from build123d import *

# Parameters (mm, degrees)
SKETCH1_R                = 7.15
SKETCH1_R_2              = 6.65
BOSS_EXTRUDE1_DEPTH      = 15
BOSS_EXTRUDE2_DEPTH      = 26.9
BOSS_EXTRUDE2_DEPTH_BACK = 11.9
SKETCH2_R                = 14
SKETCH2_R_2              = 8.9
CUT_EXTRUDE12_START      = -15
SKETCH50_R               = 14
SKETCH50_R_2             = 10.9
CUT_EXTRUDE12_DEPTH      = 10
CUT_EXTRUDE8_DEPTH       = 10
CUT_EXTRUDE8_DEPTH_BACK  = 21.28
SKETCH30_R               = 7.65
CIRPATTERN3_COUNT        = 6
BOSS_EXTRUDE3_START      = 1.2999999
BOSS_EXTRUDE3_DEPTH      = 1.6000002
CUT_EXTRUDE11_START      = 2.5
SKETCH38_R               = 11.53
CUT_EXTRUDE11_DEPTH      = 10
CUT_EXTRUDE13_DEPTH      = 39.000263325
CUT_EXTRUDE13_DEPTH_BACK = 39.000263325
SKETCH51_W               = 20.008016057
SKETCH51_H               = 32.534282003
CIRPATTERN4_COUNT        = 6
FILLET1_R                = 0.25


# Read off the part's stored shape, not the designer's step: Boss-Extrude3
with BuildPart() as part:
    # Sketch1 → Boss-Extrude1 (new body)
    with BuildSketch(Plane.XY):
        Circle(SKETCH1_R)
        Circle(SKETCH1_R_2, mode=Mode.SUBTRACT)
    extrude(amount=BOSS_EXTRUDE1_DEPTH)

    # Sketch2 → Boss-Extrude2 (add, two sides: drawn at the far end of the back side and taken through both)
    with BuildSketch(Plane(origin=(0, 0, 0), x_dir=(1, 0, 0), z_dir=(0, 1, 0)).offset(-BOSS_EXTRUDE2_DEPTH_BACK)):
        with Locations(Location((0, 8.9, 0), (0, 0, 270))):
            Circle(SKETCH2_R)
        with Locations(Location((0, 8.9, 0), (0, 0, 270))):
            Circle(SKETCH2_R_2, mode=Mode.SUBTRACT)
    extrude(amount=BOSS_EXTRUDE2_DEPTH + BOSS_EXTRUDE2_DEPTH_BACK)

    # Sketch50 → Cut-Extrude12 (cut)
    with BuildSketch(Plane(origin=(0, 26.9, 0), x_dir=(1, 0, 0), z_dir=(0, 1, 0)).offset(CUT_EXTRUDE12_START)):
        with Locations(Location((0, 8.9, 0), (0, 0, 270))):
            Circle(SKETCH50_R)
        with Locations(Location((0, 8.9, 0), (0, 0, 270))):
            Circle(SKETCH50_R_2, mode=Mode.SUBTRACT)
    extrude(amount=CUT_EXTRUDE12_DEPTH, mode=Mode.SUBTRACT)

    # Sketch30 → Cut-Extrude8 (cut, two sides: drawn at the far end of the back side and taken through both)
    with BuildSketch(Plane.XY.offset(15).offset(-CUT_EXTRUDE8_DEPTH_BACK)):
        with Locations(Location((0, 0, 0), (0, 0, 90.000000001))):
            Circle(SKETCH30_R)
    extrude(amount=CUT_EXTRUDE8_DEPTH + CUT_EXTRUDE8_DEPTH_BACK, mode=Mode.SUBTRACT)

    # Sketch47 → Tap Drill for M2 Tap1 (revolve, cut)
    with BuildSketch(Plane(origin=(0, 26.9, 2.1), x_dir=(0, 0, 1), z_dir=(1, 0, 0))):
        Polygon((0, 0), (0, 4.480688495), (0.8, 4), (0.8, 0), align=None)
    tap_drill_for_m2_tap1 = revolve(axis=Axis((0, 33.25, 2.1), (0, -1, 0)), mode=Mode.SUBTRACT)

    # CirPattern3: Tap Drill for M2 Tap1 ×6 about axis
    cirpattern3_axis = Axis((0, 0, -8.9), (0, 1, 0))
    for i in range(1, CIRPATTERN3_COUNT):
        add(tap_drill_for_m2_tap1.rotate(cirpattern3_axis, i * 360 / CIRPATTERN3_COUNT), mode=Mode.SUBTRACT)

    # Mirror1: Tap Drill for M2 Tap1 across plane
    add(tap_drill_for_m2_tap1.mirror(Plane.ZX.offset(7.5)), mode=Mode.SUBTRACT)

    # Mirror1 copy 1 sketch → Mirror1 copy 1 (revolve, cut)
    with BuildSketch(Plane(origin=(9.526279442, -11.9, -3.4), x_dir=(0.8660254037844386, 0, 0.5000000000000001), z_dir=(0.5000000000000001, 0, -0.8660254037844386))):
        Polygon((0, 0), (0, -4.480688495), (0.8, -4), (0.8, 0), align=None)
    revolve(axis=Axis((9.526279442, -18.25, -3.4), (0, -1, 0)), mode=Mode.SUBTRACT)

    # Mirror1 copy 2 sketch → Mirror1 copy 2 (revolve, cut)
    with BuildSketch(Plane(origin=(9.526279442, -11.9, -14.4), x_dir=(0.8660254037844387, 0, -0.4999999999999998), z_dir=(-0.4999999999999998, 0, -0.8660254037844387))):
        Polygon((0, 0), (0, -4.480688495), (0.8, -4), (0.8, 0), align=None)
    revolve(axis=Axis((9.526279442, -18.25, -14.4), (0, -1, 0)), mode=Mode.SUBTRACT)

    # Mirror1 copy 3 sketch → Mirror1 copy 3 (revolve, cut)
    with BuildSketch(Plane(origin=(0, -11.9, -19.9), x_dir=(0, 0, -1), z_dir=(-1, 0, 0))):
        Polygon((0, 0), (0, -4.480688495), (0.8, -4), (0.8, 0), align=None)
    revolve(axis=Axis((0, -18.25, -19.9), (0, -1, 0)), mode=Mode.SUBTRACT)

    # Mirror1 copy 4 sketch → Mirror1 copy 4 (revolve, cut)
    with BuildSketch(Plane(origin=(-9.526279442, -11.9, -14.4), x_dir=(-0.8660254037844384, 0, -0.5000000000000004), z_dir=(-0.5000000000000004, 0, 0.8660254037844384))):
        Polygon((0, 0), (0, -4.480688495), (0.8, -4), (0.8, 0), align=None)
    revolve(axis=Axis((-9.526279442, -18.25, -14.4), (0, -1, 0)), mode=Mode.SUBTRACT)

    # Mirror1 copy 5 sketch → Mirror1 copy 5 (revolve, cut)
    with BuildSketch(Plane(origin=(-9.526279442, -11.9, -3.4), x_dir=(-0.8660254037844386, 0, 0.5000000000000001), z_dir=(0.5000000000000001, 0, 0.8660254037844386))):
        Polygon((0, 0), (0, -4.480688495), (0.8, -4), (0.8, 0), align=None)
    revolve(axis=Axis((-9.526279442, -18.25, -3.4), (0, -1, 0)), mode=Mode.SUBTRACT)

    # Boss-Extrude3 outline → Boss-Extrude3 (add)
    with BuildSketch(Plane.XY.offset(BOSS_EXTRUDE3_START)):
        with BuildLine():
            Line((-2, -11.9), (2, -11.9))
            Line((2, -11.9), (2, -7.383935265))
            ThreePointArc((2, -7.383935265), (0, -7.65), (-2, -7.383935265))
            Line((-2, -7.383935265), (-2, -11.9))
        make_face()
    extrude(amount=BOSS_EXTRUDE3_DEPTH)

    # Sketch38 → Cut-Extrude11 (cut)
    with BuildSketch(Plane.XY.offset(CUT_EXTRUDE11_START)):
        Circle(SKETCH38_R)
    extrude(amount=CUT_EXTRUDE11_DEPTH, mode=Mode.SUBTRACT)

    # Sketch51 → Cut-Extrude13 (cut, two sides: drawn at the far end of the back side and taken through both)
    with BuildSketch(Plane(origin=(0, 0, 0), x_dir=(0, 0, -1), z_dir=(1, 0, 0)).offset(-CUT_EXTRUDE13_DEPTH_BACK)):
        with Locations((-12.504008029, -1.384089117)):
            Rectangle(SKETCH51_W, SKETCH51_H)
    extrude(amount=CUT_EXTRUDE13_DEPTH + CUT_EXTRUDE13_DEPTH_BACK, mode=Mode.SUBTRACT)

    # Sketch49 → Tap Drill for M1.6 Tap1 (revolve, cut)
    with BuildSketch(Plane(origin=(-5, 8.660254038, 2.5), x_dir=(0, -1, 0), z_dir=(1, 0, 0))):
        Polygon((0, 0), (0, 3.375537887), (0.625, 3), (0.625, 0), align=None)
    tap_drill_for_m1_6_tap1 = revolve(axis=Axis((-5, 8.660254038, 8.85), (0, 0, -1)), mode=Mode.SUBTRACT)

    # CirPattern4: Tap Drill for M1.6 Tap1 ×6 about axis, 2 skipped
    cirpattern4_axis = Axis((0, 0, 25), (0, 0, 1))
    add([tap_drill_for_m1_6_tap1.rotate(cirpattern4_axis, i * 360 / CIRPATTERN4_COUNT) for i in range(1, CIRPATTERN4_COUNT) if i not in (1, 4)], mode=Mode.SUBTRACT)

    # Fillet1
    fillet1_edges = [part.edges().sort_by_distance(p)[0] for p in [
        (0, 11.9, -19.8),
        (0, 21.9, -19.8),
    ]]
    fillet(fillet1_edges, radius=FILLET1_R)


solid = part.part
Verification items for the finished model (mm, model axes). A direction names the side the tool comes from. Coordinates: 2 decimals unless noted, no trailing zeros. Write each loop counter-clockwise with the first axis right and the second up, starting at its lowest first coordinate (ties: lowest second). Pieces come first, ordered by that corner, then holes. Notation, with made-up numbers: M 30,-19 L 63,-19 A12 cw 63,0 Z; hole C -36.75,-17.5 d1. An arc over 180 degrees is marked long. Use a Markdown table: item, result.
Q1. Draft check along Z on faces 6 (the face through (9.611, -7.503, -14.51)), 7 (the face through (-5.188, 8.064, 1.021)), 8 (the face through (-8.52, 24.36, -20.01)). Enter one of: +Z half, -Z half, draft (parallel to the pull), parting line (faces both ways), or undercut.
Reply:
| item | result |
|---|---|
| face 6 | undercut |
| face 7 | draft |
| face 8 | parting line |
Q2. Sectioned sample at C-C, the plane y = 0. Record the boundary of the cut face in (x, z).
Reply:
| item | result |
|---|---|
| outline | M -8.13,2.5 A14 ccw long 8.13,2.5 L 7.65,2.5 L 7.65,-4.35 A8.9 cw long -7.65,-4.35 L -7.65,2.5 Z |
Q3. Thickness scan on line 1 (Y direction, x = 11, z = -16); line 2 (X direction, y = 24.5, z = -14.4); line 3 (Y direction, x = 6.25, z = 0.75). Record the ranges inside material, lowest first.
Reply:
| item | result |
|---|---|
| line 1 | y = -11.9 to 11.9, 21.9 to 26.9 |
| line 2 | x = -12.87 to -10.33, -8.73 to -7, 7 to 8.73, 10.33 to 12.87 |
| line 3 | y = -11.9 to -4.41, 4.41 to 11.9, 21.9 to 26.9 |
Q4. Go/stop test with flat-tipped pins: P1, Ø6, axis at y = 6.5, z = -16, coming from the +X side; P2, Ø1, axis at x = 5, y = -8.66, coming from the +Z side; P3, Ø1.8, axis at x = 0, z = -19.9, coming from the -Y side; P4, Ø1.6, axis at x = -5, y = -8.66, coming from the +Z side. Record where each tip stops, or that it passes through.
Reply:
| item | result |
|---|---|
| P1 | stops at x = 13.39 |
| P2 | stops at z = -0.57 |
| P3 | stops at y = -11.9 |
| P4 | stops at z = 2.5 |
Q5. Sectioned sample at A-A, the plane z = -8.9. Record the boundary of the cut face in (x, y), plus the area to 3 significant figures.
Reply:
| item | result |
|---|---|
| outline | M -14,-11.9 L -8.9,-11.9 L -8.9,26.9 L -14,26.9 L -14,21.9 L -11.15,21.9 A0.25 cw -10.9,21.65 L -10.9,12.15 A0.25 cw -11.15,11.9 L -14,11.9 Z; M 8.9,-11.9 L 14,-11.9 L 14,11.9 L 11.15,11.9 A0.25 cw 10.9,12.15 L 10.9,21.65 A0.25 cw 11.15,21.9 L 14,21.9 L 14,26.9 L 8.9,26.9 Z |
| area | 334 mm² |
Q6. Sectioned sample at B-B, the plane y = 20. Record the boundary of the cut face in (x, z), plus the area to 3 significant figures.
Reply:
| item | result |
|---|---|
| outline | C 0,-8.9 d21.8; hole C 0,-8.9 d17.8 |
| area | 124 mm² |
Q7. Set-up check for faces 1 (the face through (-9.1, 26.9, -9.1)), 2 (the face through (-5.42, -8.2, 1.02)), 3 (the face through (-10.3, 24.9, -3.2)), 4 (the face through (10.2, -9.93, -3.83)), 5 (the face through (0.48, 16.83, -19.79)): record each of +Z, -Z, +X, -X, +Y, -Y from which the full face is reachable in a straight line by a thin tool's end or side.
Reply:
| item | result |
|---|---|
| face 1 | +Z, -Z, +X, -X, +Y |
| face 2 | +Z |
| face 3 | +Y |
| face 4 | -Y |
| face 5 | none |
